```python
from build123d import *

# Parameters (mm, degrees)
PAD005_DEPTH = 110
BOX049_W     = 117
BOX049_H     = 104
BOX049_DEPTH = 3
BOX048_W     = 118.2
BOX048_H     = 106.4
BOX048_DEPTH = 3


with BuildPart() as pad_rahmen:
    # Sketch010 → Pad005 (new body)
    with BuildSketch(Plane.XZ):
        Polygon((0, 0), (2.01, 0), (6.250278, 40.343548), (0, 40.343548), align=None)
    extrude(amount=-PAD005_DEPTH)


with BuildPart() as cube041:
    # Box049 → Box049 (new body)
    with BuildSketch(Plane(origin=(0, 1.2, 0), x_dir=(1, 0, 0), z_dir=(0, 0, 1))):
        with Locations((58.5, 52)):
            Rectangle(BOX049_W, BOX049_H)
    extrude(amount=BOX049_DEPTH)


with BuildPart() as rahmen_cut:
    # Box048 → Box048 (new body)
    with BuildSketch(Plane.XY):
        with Locations((59.1, 53.2)):
            Rectangle(BOX048_W, BOX048_H)
    extrude(amount=BOX048_DEPTH)

    # Cut048: cut Cube041
    add(cube041.part, mode=Mode.SUBTRACT)


with BuildPart() as rahmen_cut_1:
    # Cut048 placement: moved
    add(rahmen_cut.part.moved(Location((0, 1.8, 20))))

    # Cut049: cut Pad_Rahmen
    add(pad_rahmen.part, mode=Mode.SUBTRACT)


solid = rahmen_cut_1.part
```
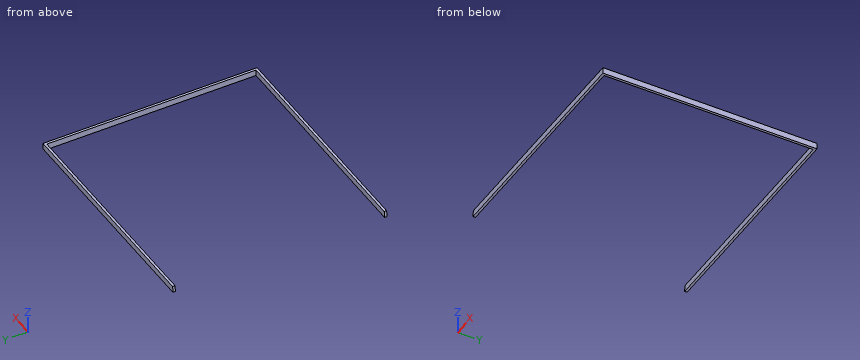
Verification items for the finished model (mm, model axes). Give positions to 0.01 mm unless a question says otherwise; leave off trailing zeros. Order: outer loops, then holes, each group sorted by start corner. A loop starts at its lowest first (then second) coordinate and runs counter-clockwise, first axis right, second up. Notation, with made-up numbers: (-19.75, -7) - (-1.75, -7) arc R15 ccw to (-1.75, -3) - close; hole circle Ø1 at (9.25, 47). An arc over 180 degrees is marked (long way). Answer as CSV lines item,"result". Start each with the question number.
Item 1: Material ranges on L1, parallel to Y at x = 43.5, z = 22; L2, parallel to X at y = 103, z = 20.75, recorded low to high.
Item 2: Section check C-C, the plane y = 30.5. Record the boundary of the cut face in (x, z), plus the area to 3 significant figures.
Item 3: Gauge pin test, flat end, axial feed: pin 1 (0.9 mm diameter, centred on y = 75.5, z = 21, fed in from -X). Record the tip position at first contact, or that the pin passes through.
Item 4: Section check B-B, the plane z = 21.75. Record the boundary of the cut face in (x, y).
Item 5: Section check A-A, the plane x = 111.5. Record the boundary of the cut face in (y, z).
Filled in:
1,L1,"1.8 to 3, 107 to 108.2"
1,L2,"117 to 118.2"
2,outline,"(117, 20) - (118.2, 20) - (118.2, 23) - (117, 23) - close"
2,area,"3.60 mm^2"
3,pin 1,"x = 117"
4,outline,"(4.3, 1.8) - (118.2, 1.8) - (118.2, 108.2) - (4.3, 108.2) - (4.3, 107) - (117, 107) - (117, 3) - (4.3, 3) - close"
5,outline,"(1.8, 20) - (3, 20) - (3, 23) - (1.8, 23) - close; (107, 20) - (108.2, 20) - (108.2, 23) - (107, 23) - close"
